The listing builds one solid part. Answer for the finished solid, in the listing's coordinates (mm). A direction names the side the tool comes from. Give positions to 0.01 mm unless a question says otherwise; leave off trailing zeros. Order: outer loops, then holes, each group sorted by start corner. A loop starts at its lowest first (then second) coordinate and runs counter-clockwise, first axis right, second up. Notation, with made-up numbers: (50, 34) - (92, 34) arc R23 cw to (92, 72) - close; hole circle Ø3 at (75.25, 14.25). An arc over 180 degrees is marked (long way). Answer as CSV lines item,"result". Start each with the question number.
1. Which of the six approach directions +Z, -Z, +X, -X, +Y, -Y give full straight-line access (tool end or side, diameter ignored) to faces 1 (the flat face through (4, 50, 27)), 2 (the flat face through (0, 1, 26))?
2. Consider line 1 along Y through (x, z) = (22, 13.25); line 2 along X through (y, z) = (19, 14); line 3 along X through (y, z) = (44, 19). Determine where each line is inside the solid, lowest interval first. Write a range as [from, to].
3. Determine the mould class of faces 3 (the cylindrical face through (0.561, 0.493, 25.494)), 4 (the cylindrical face through (0.627, 24.65, 28.493)), 5 (the cylindrical face through (0.594, 25.157, 26.993)), 6 (the flat face through (28, 25, 0)) for opening direction X: +X half, -X half, draft (parallel to the pull), parting line (faces both ways), or undercut.
4. Section B-B on x = 0 is taken. Give the vertices of the cut face in (y, z).
5. Section C-C on y = 46.5 is taken. Give the vertices of the cut face in (x, z).
6. Flat-ended cylindrical pins translate along their axes: pin 1 (1 mm diameter, centred on y = 42.5, z = 14.5, fed in from +X); pin 2 (1.5 mm diameter, centred on x = 22, y = 43.5, fed in from -Z); pin 3 (2 mm diameter, centred on y = 5.5, z = 8.5, fed in from -X). Find the tip coordinate at first contact, or state that the pin passes through.
7. Section D-D on z = 5 is taken. Give the vertices of the cut face in (x, y) (3 decimals), and give its area (3 significant figures).
8. Section A-A on z = 15 is taken. Give the vertices of the cut face in (x, y), and give its area (3 significant figures).
from build123d import *

# Parameters (mm, degrees)
PAD_DEPTH    = 50
PAD001_DEPTH = 1


with BuildPart() as part:
    # Sketch → Pad (new body)
    with BuildSketch(Plane.XZ):
        with BuildLine():
            ThreePointArc((28.5, 0), (0, 28.5), (-28.5, 0))
            Line((-28.5, 0), (-27, 0))
            ThreePointArc((27, 0), (0, 27), (-27, 0))
            Line((27, 0), (28.5, 0))
        make_face()
    extrude(amount=-PAD_DEPTH)

    # Sketch001 → Pad001 (join)
    with BuildSketch(Plane.XZ):
        with BuildLine():
            ThreePointArc((28.5, 0), (0, 28.5), (-28.5, 0))
            Line((-28.5, 0), (-25.5, 0))
            ThreePointArc((25.5, 0), (0, 25.5), (-25.5, 0))
            Line((25.5, 0), (28.5, 0))
        make_face()
    extrude(amount=-PAD001_DEPTH)


solid = part.part
Checks:
1,face 1,"+Z, -Z, +X, -X, +Y"
1,face 2,"-Z, +Y"
2,line 1,"y = [0, 1]"
2,line 2,"x = [-24.82, -23.09], [23.09, 24.82]"
2,line 3,"x = [-21.24, -19.18], [19.18, 21.24]"
3,face 3,"undercut"
3,face 4,"parting line"
3,face 5,"undercut"
3,face 6,"draft"
4,outline,"(0, 25.5) - (1, 25.5) - (1, 27) - (50, 27) - (50, 28.5) - (0, 28.5) - close"
5,outline,"(-28.5, 0) - (-27, 0) arc R27 cw to (27, 0) - (28.5, 0) arc R28.5 ccw to start"
6,pin 1,"stops at x = 24.82"
6,pin 2,"stops at z = 14.54"
6,pin 3,"stops at x = -27.5"
7,outline,"(-28.058, 0) - (-25.005, 0) - (-25.005, 1) - (-26.533, 1) - (-26.533, 50) - (-28.058, 50) - close; (25.005, 0) - (28.058, 0) - (28.058, 50) - (26.533, 50) - (26.533, 1) - (25.005, 1) - close"
7,area,"156 mm²"
8,outline,"(-24.23, 0) - (-20.62, 0) - (-20.62, 1) - (-22.45, 1) - (-22.45, 50) - (-24.23, 50) - close; (20.62, 0) - (24.23, 0) - (24.23, 50) - (22.45, 50) - (22.45, 1) - (20.62, 1) - close"
8,area,"182 mm²"
